from build123d import *

# Parameters (mm, degrees)
SKETCH3_W           = 122.1
SKETCH3_H           = 197.8
BOSS_EXTRUDE2_DEPTH = 3
SKETCH4_R           = 7.5
CUT_EXTRUDE2_DEPTH  = 3
SKETCH5_W           = 185.639017853
SKETCH5_H           = 93.814581834
CUT_EXTRUDE3_DEPTH  = 12
SKETCH7_W           = 181.97184254
SKETCH7_H           = 161.609726855
CUT_EXTRUDE4_DEPTH  = 19
CUT_EXTRUDE8_DEPTH  = 10
SKETCH10_W          = 122.1
SKETCH10_H          = 3
BOSS_EXTRUDE3_DEPTH = 18.6


with BuildPart() as part:
    # Sketch3 → Boss-Extrude2 (new body)
    with BuildSketch(Plane(origin=(0, 0, 0), x_dir=(1, 0, 0), z_dir=(0, 1, 0))):
        with Locations((61.05, 98.9)):
            Rectangle(SKETCH3_W, SKETCH3_H)
    extrude(amount=BOSS_EXTRUDE2_DEPTH)

    # Sketch4 → Cut-Extrude2 (cut)
    with BuildSketch(Plane(origin=(0, 3, 0), x_dir=(1, 0, 0), z_dir=(0, 1, 0))):
        with Locations((16.92, 152.8)):
            Circle(SKETCH4_R)
        with Locations((105.18, 152.8)):
            Circle(SKETCH4_R)
        with BuildLine():
            Line((20.17, 145.3), (20.17, 45.3))
            ThreePointArc((20.17, 45.3), (16.92, 42.05), (13.67, 45.3))
            Line((13.67, 45.3), (13.67, 145.3))
            ThreePointArc((13.67, 145.3), (16.92, 148.55), (20.17, 145.3))
        make_face()
        with BuildLine():
            Line((101.93, 145.3), (101.93, 45.3))
            ThreePointArc((101.93, 45.3), (105.18, 42.05), (108.43, 45.3))
            Line((108.43, 45.3), (108.43, 145.3))
            ThreePointArc((108.43, 145.3), (105.18, 148.55), (101.93, 145.3))
        make_face()
    extrude(amount=-CUT_EXTRUDE2_DEPTH, mode=Mode.SUBTRACT)

    # Sketch5 → Cut-Extrude3 (cut)
    with BuildSketch(Plane(origin=(0, 0, -197.8), x_dir=(-1, 0, 0), z_dir=(0, 0, -1))):
        with Locations((-62.393879106, -6.143731482)):
            Rectangle(SKETCH5_W, SKETCH5_H)
    extrude(amount=-CUT_EXTRUDE3_DEPTH, mode=Mode.SUBTRACT)

    # Sketch7 → Cut-Extrude4 (cut)
    with BuildSketch(Plane.XY):
        with Locations((66.543858185, 9.384028943)):
            Rectangle(SKETCH7_W, SKETCH7_H)
    extrude(amount=-CUT_EXTRUDE4_DEPTH, mode=Mode.SUBTRACT)

    # Sketch8 → Cut-Extrude8 (cut)
    with BuildSketch(Plane(origin=(0, 3, 0), x_dir=(1, 0, 0), z_dir=(0, 1, 0))):
        with BuildLine():
            ThreePointArc((13.67, 106.308017417), (16.91951533, 105.565143685), (20.17, 106.303764471))
            Line((20.17, 106.303764471), (20.17, 145.3))
            ThreePointArc((20.17, 145.3), (20.150641933, 145.654193023), (20.09279834, 146.004166667))
            ThreePointArc((20.09279834, 146.004166667), (21.056311174, 159.056271243), (9.424422573, 153.057524837))
            Line((9.424422573, 153.057524837), (9.424422573, 152.542475163))
            ThreePointArc((9.424422573, 152.542475163), (10.663728757, 148.663688826), (13.74720166, 146.004166667))
            ThreePointArc((13.74720166, 146.004166667), (13.689358067, 145.654193023), (13.67, 145.3))
            Line((13.67, 145.3), (13.67, 106.308017417))
        make_face()
        with BuildLine():
            ThreePointArc((112.675577427, 153.06514208), (105.175577427, 160.56514208), (97.675577427, 153.06514208))
            Line((97.675577427, 153.06514208), (97.675577427, 113.06514208))
            ThreePointArc((97.675577427, 113.06514208), (98.827671051, 109.070885622), (101.93, 106.303764471))
            Line((101.93, 106.303764471), (101.93, 145.3))
            ThreePointArc((101.93, 145.3), (101.949358067, 145.654193023), (102.00720166, 146.004166667))
            ThreePointArc((102.00720166, 146.004166667), (101.043688826, 159.056271243), (112.675577427, 153.057524837))
            Line((112.675577427, 153.057524837), (112.675577427, 153.06514208))
        make_face()
        with BuildLine():
            Line((108.43, 145.3), (108.43, 106.308017417))
            ThreePointArc((108.43, 106.308017417), (111.526095882, 109.075039907), (112.675577427, 113.06514208))
            Line((112.675577427, 113.06514208), (112.675577427, 152.542475163))
            ThreePointArc((112.675577427, 152.542475163), (111.436271243, 148.663688826), (108.35279834, 146.004166667))
            ThreePointArc((108.35279834, 146.004166667), (108.410641933, 145.654193023), (108.43, 145.3))
        make_face()
        with BuildLine():
            ThreePointArc((9.424422573, 113.06514208), (10.573904118, 109.075039907), (13.67, 106.308017417))
            Line((13.67, 106.308017417), (13.67, 145.3))
            ThreePointArc((13.67, 145.3), (13.689358067, 145.654193023), (13.74720166, 146.004166667))
            ThreePointArc((13.74720166, 146.004166667), (10.663728757, 148.663688826), (9.424422573, 152.542475163))
            Line((9.424422573, 152.542475163), (9.424422573, 113.06514208))
        make_face()
        with BuildLine():
            Line((24.424422573, 113.06514208), (24.424422573, 153.06514208))
            ThreePointArc((24.424422573, 153.06514208), (16.924422573, 160.56514208), (9.424422573, 153.06514208))
            Line((9.424422573, 153.06514208), (9.424422573, 153.057524837))
            ThreePointArc((9.424422573, 153.057524837), (21.056311174, 159.056271243), (20.09279834, 146.004166667))
            ThreePointArc((20.09279834, 146.004166667), (20.150641933, 145.654193023), (20.17, 145.3))
            Line((20.17, 145.3), (20.17, 106.303764471))
            ThreePointArc((20.17, 106.303764471), (23.272328949, 109.070885622), (24.424422573, 113.06514208))
        make_face()
    extrude(amount=-CUT_EXTRUDE8_DEPTH, mode=Mode.SUBTRACT)

    # Sketch10 → Boss-Extrude3 (add)
    with BuildSketch(Plane.XY.offset(-19)):
        with Locations((61.05, 1.5)):
            Rectangle(SKETCH10_W, SKETCH10_H)
    extrude(amount=BOSS_EXTRUDE3_DEPTH)


solid = part.part
Input: part model. Units: mm. Frame: model coordinates. A direction names the side the tool comes from. Give positions to 0.01 mm unless a question says otherwise; leave off trailing zeros. Write each loop counter-clockwise with the first axis right and the second up, starting at its lowest first coordinate (ties: lowest second). Pieces come first, ordered by that corner, then holes. Notation, with made-up numbers: M 68,39 L 87,39 A34 cw 87,73 Z; hole C -6.75,-15 d6. An arc over 180 degrees is marked long. Write item = value, one per line. Start each with the question number.
1) Cut plane B-B on x = 105.18. Return the cut outline in (y, z).
2) First-contact query: pin 1 Ø8 at (x, z) = (106.5, -125) entering from +Y. Flat tip, straight axial feed; report the tip coordinate or a pass-through.
3) Reachability of faces 1 (the flat face through (60, 0, -94)), 2 (the cylindrical face through (23.24, 1.52, -109.02)) from +Z, -Z, +X, -X, +Y, -Y: full face, straight path, thin tool, end or side. Return the list, or none.
4) Cut plane D-D on x = 17. Return the cut outline in (y, z).
5) Cut plane C-C on z = -135.5. Return the cut outline in (x, y), then the cut area to 3 significant figures.
6) Draft query along Z for faces 3 (the cylindrical face through (17.089, 1.521, -160.563)), 4 (the flat face through (60, 3, -94)). Return one class per face: +Z half, -Z half, draft (parallel to the pull), parting line (faces both ways), or undercut.
7) Material intervals for line 1 along X through (y, z) = (2.9, -58); line 2 along X through (y, z) = (1.3, -128.5); line 3 along Z through (x, y) = (23, 1.45), sorted ascending. Write a range as [from, to].
8) Cut plane A-A on y = 2.45. Count the separate pieces of the cut face and the enclosed holes in it, then the cut area to 3 significant figures.
Solved:
q1.outline = M 0,-185.8 L 3,-185.8 L 3,-160.57 L 0,-160.57 Z; M 0,-42.05 L 3,-42.05 L 3,-0.4 L 0,-0.4 Z
q2.pin_1 = through
q3.face_1 = +Z, -Z, +X, -X, -Y
q3.face_2 = +Y, -Y
q4.outline = M 0,-185.8 L 3,-185.8 L 3,-160.56 L 0,-160.56 Z; M 0,-42.05 L 3,-42.05 L 3,-0.4 L 0,-0.4 Z
q5.outline = M 0,0 L 9.42,0 L 9.42,3 L 0,3 Z; M 24.42,0 L 97.68,0 L 97.68,3 L 24.42,3 Z; M 112.68,0 L 122.1,0 L 122.1,3 L 112.68,3 Z
q5.area = 276 mm2
q6.face_3 = undercut
q6.face_4 = draft
q7.line_1 = [0, 13.67], [20.17, 101.93], [108.43, 122.1]
q7.line_2 = [0, 9.42], [24.42, 97.68], [112.68, 122.1]
q7.line_3 = [-185.8, -157.46], [-108.67, -0.4]
q8.separate_pieces = 1
q8.enclosed_holes = 2
q8.area = 20,300 mm2
